Could you check a few things on this model? Use its own coordinates, in mm. Face numbers are marked on the shaded views. A direction names the side the tool comes from. Round coordinates to 2 decimals unless told otherwise and drop trailing zeros. Write each loop counter-clockwise with the first axis right and the second up, starting at its lowest first coordinate (ties: lowest second). Pieces come first, ordered by that corner, then holes. Notation, with made-up numbers: (54, 75) - (90, 75) arc R24 cw to (90, 113) - close; hole circle Ø2 at (39.25, 14). An arc over 180 degrees is marked (long way). Write each question's results on one line, items separated by ' | '. Start each with the question number.
(1) Please list where these lines run through material, in increasing order: line 1 (X direction, y = 0, z = 0.65); line 2 (Z direction, x = -18.5, y = 4.25); line 3 (Z direction, x = 24.5, y = -3.75). Write a range as [from, to].
(2) Imagine slicing it at C-C on x = -17. Write out the boundary of the cut face in (y, z).
(3) For P1, Ø1.2, axis at x = -14, y = 2.5, coming from the +Z side; P2, Ø1, axis at x = -16.5, y = -3.5, coming from the +Z side; P3, Ø5, axis at x = -2, y = -1.5, coming from the +Z side, each with a flat end and sliding along its axis, tell me the tip position at first contact or that it passes through.
(4) Imagine slicing it at A-A on y = 0.25. Write out the boundary of the cut face in (x, z), then the cut area to 3 significant figures.
(5) Thinking about a two-plate mould opening in X: for the marked faces 1 and 2, which applies, +X half, -X half, draft (parallel to the pull), parting line (faces both ways), or undercut?
(6) Imagine slicing it at B-B on x = 1. Write out the boundary of the cut face in (y, z), then the cut area to 3 significant figures.
(7) On a 3-axis mill with a long thin cutter (end or side, diameter ignored), from which of +Z, -Z, +X, -X, +Y, -Y can I reach the whole of each face in a straight line? I mean the marked faces 3, 4 and 5. Say none if no direction works.
```python
from build123d import *

# Parameters (mm, degrees)
F0_W      = 60
F0_H      = 10
F1_DEPTH  = 0.2
F2_W      = 25
F2_H      = 10
F3_DEPTH  = 0.1
F4_W      = 1.5
F4_H      = 10
F5_DEPTH  = 0.3
F6_W      = 10.5
F6_H      = 10
F7_DEPTH  = 0.3
F8_W      = 7
F8_H      = 10
F9_DEPTH  = 0.7
F10_W     = 8
F10_H     = 10
F11_DEPTH = 0.7
F12_W     = 17.5
F12_H     = 10
F13_DEPTH = 1.2
F14_W     = 2.5
F14_H     = 10
F15_DEPTH = 1.2


with BuildPart() as f1:
    # F0 (on Top) → F1 (new body)
    with BuildSketch(Plane.XY):
        Rectangle(F0_W, F0_H)
    extrude(amount=F1_DEPTH)

    # F2 (on face) → F3 (join)
    with BuildSketch(Plane.XY.offset(0.2)):
        Rectangle(F2_W, F2_H)
    extrude(amount=F3_DEPTH)

    # F4 (on face) → F5 (join)
    with BuildSketch(Plane.XY.offset(0.3)):
        with Locations((-11.75, 0)):
            Rectangle(F4_W, F4_H)
    extrude(amount=F5_DEPTH)

    # F6 (on face) → F7 (join)
    with BuildSketch(Plane.XY.offset(0.2)):
        with Locations((-17.75, 0)):
            Rectangle(F6_W, F6_H)
    extrude(amount=F7_DEPTH)

    # F8 (on face) → F9 (join)
    with BuildSketch(Plane.XY.offset(0.2)):
        with Locations((-26.5, 0)):
            Rectangle(F8_W, F8_H)
    extrude(amount=F9_DEPTH)

    # F10 (on face) → F11 (join)
    with BuildSketch(Plane.XY.offset(0.5)):
        with Locations((-19, 0)):
            Rectangle(F10_W, F10_H)
    extrude(amount=F11_DEPTH)

    # F12 (on face) → F13 (join)
    with BuildSketch(Plane.XY.offset(0.2)):
        with Locations((21.25, 0)):
            Rectangle(F12_W, F12_H)
    extrude(amount=F13_DEPTH)

    # F14 (on face) → F15 (join)
    with BuildSketch(Plane.XY.offset(0.3)):
        with Locations((11.25, 0)):
            Rectangle(F14_W, F14_H)
    extrude(amount=F15_DEPTH)


solid = f1.part
```
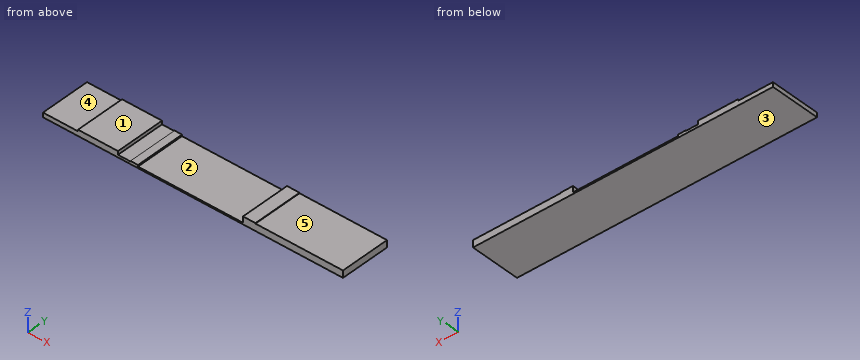
Response:
1) line 1: [-30, -15], [10, 30] | line 2: [0, 1.2] | line 3: [0, 1.4]
2) outline: (-5, 0) - (5, 0) - (5, 1.2) - (-5, 1.2) - close
3) P1: z = 0.5 | P2: z = 1.2 | P3: z = 0.3
4) outline: (-30, 0) - (30, 0) - (30, 1.4) - (12.5, 1.4) - (12.5, 1.5) - (10, 1.5) - (10, 0.3) - (-11, 0.3) - (-11, 0.6) - (-12.5, 0.6) - (-12.5, 0.5) - (-15, 0.5) - (-15, 1.2) - (-23, 1.2) - (-23, 0.9) - (-30, 0.9) - close | area: 52.6 mm²
5) face 1: draft | face 2: undercut
6) outline: (-5, 0) - (5, 0) - (5, 0.3) - (-5, 0.3) - close | area: 3.00 mm²
7) face 3: -Z, +X, -X, +Y, -Y | face 4: +Z, -X, +Y, -Y | face 5: +Z, +X, +Y, -Y
